Design review of the part shown in the three views and the two pictorial views. Dimensions are in mm from the part's minimum x, y and z. Coordinates: 2 decimals unless noted, no trailing zeros. Loops run counter-clockwise (first coordinate to the right, second up) from the corner with the lowest first, then second, coordinate; pieces in that order, holes last. Notation, with made-up numbers: (1, 48.25) -> (9, 48.25) arc R20 ccw to (9, 59.25) -> close; hole circle Ø6 at (23.25, -9). An arc over 180 degrees is marked (long way). One line per item, written item: value.
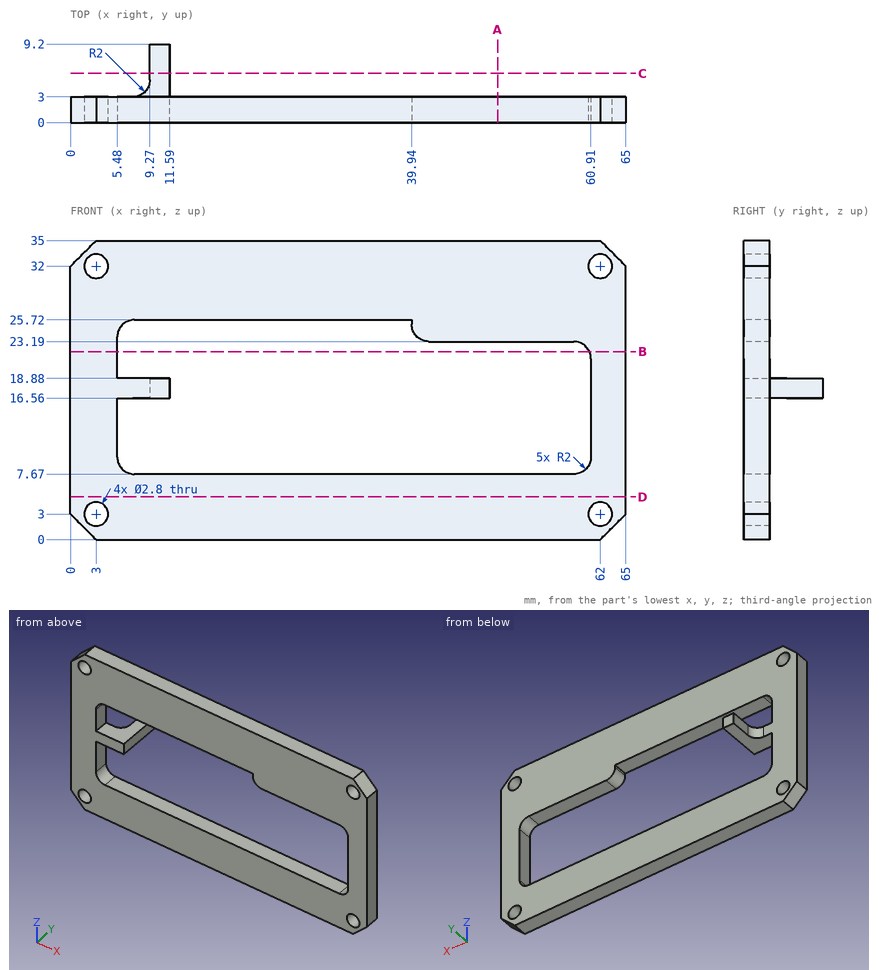
1. Take a section at B-B, the plane z = 22. Give the boundary of the cut face in (x, y).
Return value:
outline: (0, 0) -> (5.48, 0) -> (5.48, 3) -> (0, 3) -> close; (60.74, 0) -> (65, 0) -> (65, 3) -> (60.74, 3) -> close
2. Insertion check: pin 1 Ø0.7 at (y, z) = (7, 18) entering from -X; pin 2 Ø8 at (x, z) = (54, 26.5) entering from +Y; pin 3 Ø2.5 at (y, z) = (6.5, 17.5) entering from +X; pin 4 Ø5 at (x, y) = (9, 5) entering from -Z. Each pin has a flat end and moves straight along its axis. Give the tip position at first contact, or say it passes through.
Return value:
pin 1: stops at x = 9.27
pin 2: stops at y = 3
pin 3: stops at x = 11.59
pin 4: stops at z = 0
3. Take a section at A-A, the plane x = 50. Give the boundary of the cut face in (y, z).
Return value:
outline: (0, 0) -> (3, 0) -> (3, 7.67) -> (0, 7.67) -> close; (0, 23.19) -> (3, 23.19) -> (3, 35) -> (0, 35) -> close
4. Take a section at D-D, the plane z = 5. Give the boundary of the cut face in (x, y), and give its area (3 significant figures).
Return value:
outline: (0, 0) -> (65, 0) -> (65, 3) -> (0, 3) -> close
area: 195 mm2
5. To check wall thickness, follow probe 1 along X at (y, z) = (1.1, 32); probe 2 along Z at (x, y) = (8, 2.5); probe 3 along Z at (x, y) = (62, 1.4). State the ranges of each line that lie inside material, in increasing order. Write a range as from..to.
Return value:
probe 1: x = 0..1.6, 4.4..60.6, 63.4..65
probe 2: z = 0..7.67, 16.56..18.88, 25.72..35
probe 3: z = 0..1.6, 4.4..30.6, 33.4..35
6. Take a section at C-C, the plane y = 5.75. Give the boundary of the cut face in (x, z), and give its area (3 significant figures).
Return value:
outline: (9.27, 16.56) -> (11.59, 16.56) -> (11.59, 18.88) -> (9.27, 18.88) -> close
area: 5.38 mm2
